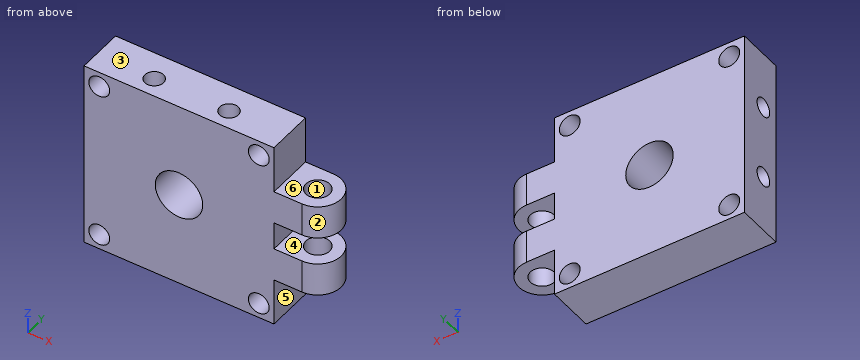
from build123d import *

# Parameters (mm, degrees)
SKETCH1_W           = 50.8
SKETCH1_H           = 50.8
SKETCH1_R           = 2.794
SKETCH1_R_2         = 6.35
BOSS_EXTRUDE1_DEPTH = 12.5
SKETCH4_R           = 3.175
BOSS_EXTRUDE2_DEPTH = 12.7
SKETCH5_W           = 13.75
SKETCH5_H           = 7.5
CUT_EXTRUDE2_DEPTH  = 13.5
SKETCH14_R          = 2.5
CUT_EXTRUDE7_DEPTH  = 20
SKETCH15_R          = 2.5
CUT_EXTRUDE8_DEPTH  = 20


with BuildPart() as part:
    # Sketch1 → Boss-Extrude1 (new body)
    with BuildSketch(Plane(origin=(0, 0, 0), x_dir=(1, 0, 0), z_dir=(0, 1, 0))):
        Rectangle(SKETCH1_W, SKETCH1_H)
        with Locations((-21.336, -21.336)):
            Circle(SKETCH1_R, mode=Mode.SUBTRACT)
        with Locations((21.336, -21.336)):
            Circle(SKETCH1_R, mode=Mode.SUBTRACT)
        with Locations((21.336, 21.336)):
            Circle(SKETCH1_R, mode=Mode.SUBTRACT)
        with Locations((-21.336, 21.336)):
            Circle(SKETCH1_R, mode=Mode.SUBTRACT)
        Circle(SKETCH1_R_2, mode=Mode.SUBTRACT)
    extrude(amount=BOSS_EXTRUDE1_DEPTH)

    # Sketch4 → Boss-Extrude2 (add, symmetric)
    with BuildSketch(Plane.XY):
        with BuildLine():
            Line((25.4, 0), (32.9, 0))
            ThreePointArc((32.9, 0), (39.15, 6.25), (32.9, 12.5))
            Line((32.9, 12.5), (25.4, 12.5))
            Line((25.4, 12.5), (25.4, 0))
        make_face()
        with Locations((32.9, 6.25)):
            Circle(SKETCH4_R, mode=Mode.SUBTRACT)
    extrude(amount=BOSS_EXTRUDE2_DEPTH, both=True)

    # Sketch5 → Cut-Extrude2 (cut, through all)
    with BuildSketch(Plane(origin=(0, 12.5, 0), x_dir=(1, 0, 0), z_dir=(0, 1, 0))):
        with Locations((32.275, 0)):
            Rectangle(SKETCH5_W, SKETCH5_H)
    extrude(amount=-CUT_EXTRUDE2_DEPTH, mode=Mode.SUBTRACT)

    # Sketch14 → Cut-Extrude7 (cut)
    with BuildSketch(Plane.XY.offset(25.4)):
        with Locations((-10, 5)):
            Circle(SKETCH14_R)
        with Locations((10, 5)):
            Circle(SKETCH14_R)
    extrude(amount=-CUT_EXTRUDE7_DEPTH, mode=Mode.SUBTRACT)

    # Sketch15 → Cut-Extrude8 (cut)
    with BuildSketch(Plane.ZY.offset(25.4)):
        with Locations((-10, 5)):
            Circle(SKETCH15_R)
        with Locations((10, 5)):
            Circle(SKETCH15_R)
    extrude(amount=-CUT_EXTRUDE8_DEPTH, mode=Mode.SUBTRACT)


solid = part.part
Model file for the job. Use its own axes, mm. Face numbers are marked on the shaded views. A direction names the side the tool comes from. Coordinates: 2 decimals unless noted, no trailing zeros. Order: outer loops, then holes, each group sorted by start corner. A loop starts at its lowest first (then second) coordinate and runs counter-clockwise, first axis right, second up. Notation, with made-up numbers: M 73.25,63 L 112.25,63 A24 ccw 112.25,90 Z; hole C 75,-35.75 d3. An arc over 180 degrees is marked long. Return JSON: item names as keys, results as strings.
1. Saw through at B-B (x = 0). Give the cut face in (y, z).
Ans:
{"outline": "M 0,-25.4 L 12.5,-25.4 L 12.5,-6.35 L 0,-6.35 Z; M 0,6.35 L 12.5,6.35 L 12.5,25.4 L 0,25.4 Z"}
2. Saw through at C-C (z = -10). Give the cut face in (x, y) (3 decimals), and give its area (3 significant figures).
Ans:
{"outline": "M -25.4,0 L 32.9,0 A6.25 ccw 32.9,12.5 L -25.4,12.5 L -25.4,7.5 L -5.4,7.5 L -5.4,2.5 L -25.4,2.5 Z; hole C 32.9,6.25 d6.35", "area": "658 mm^2"}
3. Flat gauge pins, fed straight in: pin 1 (1 mm diameter, centred on x = 32, y = 9.5, fed in from -Z); pin 2 (5 mm diameter, centred on y = 4, z = 17, fed in from +X); pin 3 (10 mm diameter, centred on x = 0, z = 0, fed in from -Y); pin 4 (1 mm diameter, centred on x = 11, y = 5.5, fed in from +Z). Where does each tip first touch, or does it go through?
Ans:
{"pin 1": "z = -12.7", "pin 2": "x = 25.4", "pin 3": "through", "pin 4": "z = 5.4"}
4. Saw through at D-D (x = 23). Give the cut face in (y, z), and give its area (3 significant figures).
Ans:
{"outline": "M 0,-25.4 L 12.5,-25.4 L 12.5,-23.58 L 0,-23.58 Z; M 0,-19.09 L 12.5,-19.09 L 12.5,19.09 L 0,19.09 Z; M 0,23.58 L 12.5,23.58 L 12.5,25.4 L 0,25.4 Z", "area": "523 mm^2"}
5. Saw through at A-A (z = 0). Give the cut face in (x, y).
Ans:
{"outline": "M -25.4,0 L -6.35,0 L -6.35,12.5 L -25.4,12.5 Z; M 6.35,0 L 25.4,0 L 25.4,12.5 L 6.35,12.5 Z"}
6. Drill centre lines: probe 1 along X at (y, z) = (7.5, 0); probe 2 along Y at (x, z) = (10, 6.5). Where is each one in solid material? Low to high.
Ans:
{"probe 1": "-25.4 to -6.35, 6.35 to 25.4", "probe 2": "0 to 2.5, 7.5 to 12.5"}
7. Tool access for the marked faces 4, 5 and 6: list every direction of +Z, -Z, +X, -X, +Y, -Y with a clear straight run to the whole face (end or side of a thin tool).
Ans:
{"face 4": "+X, +Y, -Y", "face 5": "-Z, +X, +Y, -Y", "face 6": "+Z, +X, +Y, -Y"}
8. Pull direction Y, two halves, no side cores. Call the marked faces 1, 2 and 3: +Y half, -Y half, draft (parallel to the pull), parting line (faces both ways), or undercut.
Ans:
{"face 1": "undercut", "face 2": "parting line", "face 3": "draft"}
